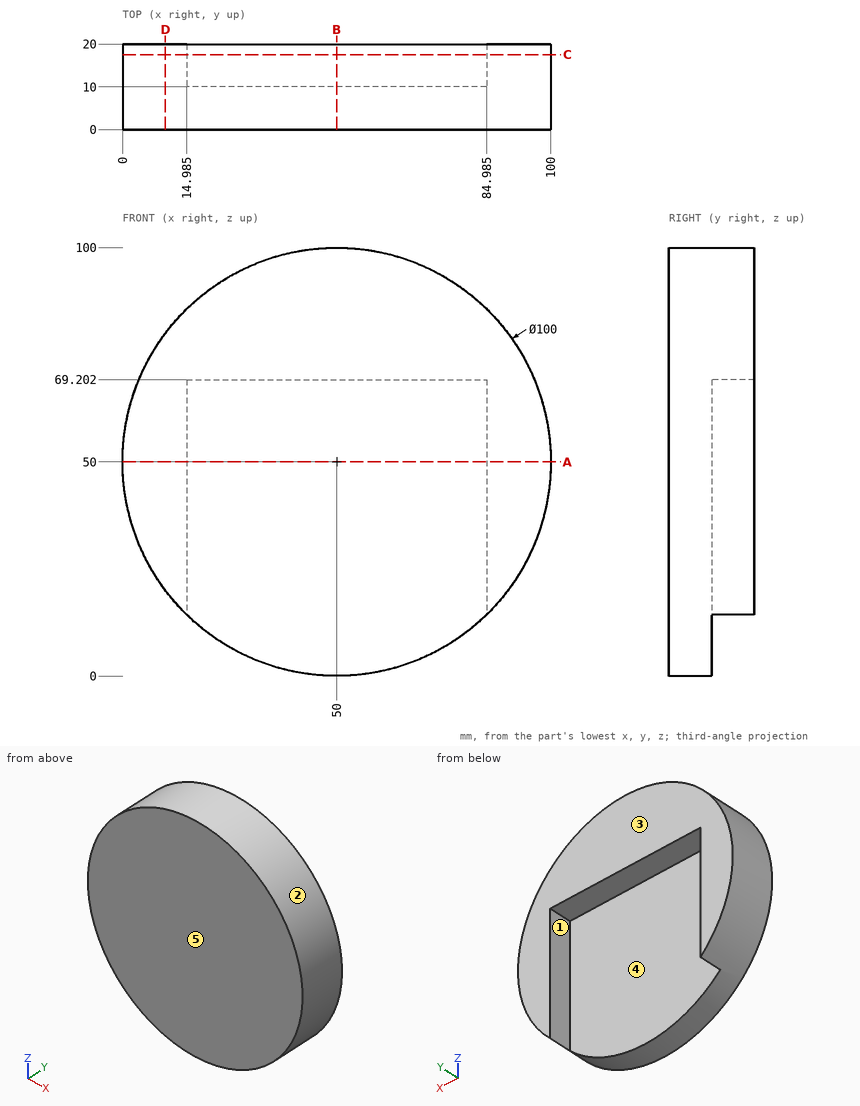
Verification items for this drawing (mm, ordinates from the low corner). A direction names the side the tool comes from. Round coordinates to 2 decimals unless told otherwise and drop trailing zeros. Loops run counter-clockwise (first coordinate to the right, second up) from the corner with the lowest first, then second, coordinate; pieces in that order, holes last. Notation, with made-up numbers: (82.25, 8) -> (98.25, 8) arc R10 ccw to (98.25, 16) -> close; hole circle Ø10 at (40.5, 83.25). An arc over 180 degrees is marked (long way). Write item = value, one per line. Start each with the question number.
1) Thickness scan on probe 1 along Y at (x, z) = (71, 34); probe 2 along X at (y, z) = (12.25, 17.5) (1 decimal); probe 3 along X at (y, z) = (5.75, 47.5). Record the ranges inside material, lowest first.
2) Sectioned sample at A-A, the plane z = 50. Record the cut outline in (x, y) (1 decimal), plus the area to 3 significant figures.
3) Gauge pin test, flat ends, axial feed: pin 1 Ø3 at (y, z) = (15, 45.5) entering from +X; pin 2 Ø8 at (y, z) = (14, 41.5) entering from -X; pin 3 Ø4 at (x, y) = (11, 15) entering from +Z. Record the tip position at first contact, or that the pin passes through.
4) Set-up check for the marked faces 4 and 5: record each of +Z, -Z, +X, -X, +Y, -Y from which the full face is reachable in a straight line by a thin tool's end or side.
5) Sectioned sample at D-D, the plane x = 10. Record the cut outline in (y, z).
6) Sectioned sample at C-C, the plane y = 17.5. Record the cut outline in (x, z) (1 decimal), plus the area to 3 significant figures.
7) Sectioned sample at B-B, the plane x = 50. Record the cut outline in (y, z), plus the area to 3 significant figures.
8) Release check for a two-part mould opening along X. For the marked faces 1, 2 and 3 record: released by +X, released by -X, zero draft, split by the parting line, or undercut.
Results are:
q1.probe_1 = 0 to 10
q1.probe_2 = 12 to 15, 85 to 88
q1.probe_3 = 0.06 to 99.94
q2.outline = (0, 0) -> (100, 0) -> (100, 20) -> (85, 20) -> (85, 10) -> (15, 10) -> (15, 20) -> (0, 20) -> close
q2.area = 1,300 mm^2
q3.pin_1 = 99.91
q3.pin_2 = 0.2
q3.pin_3 = 83.63
q4.face_4 = -Z, +Y
q4.face_5 = +Z, -Z, +X, -X, -Y
q5.outline = (0, 20) -> (20, 20) -> (20, 80) -> (0, 80) -> close
q6.outline = (15, 14.3) -> (15, 69.2) -> (85, 69.2) -> (85, 14.3) arc R50 ccw (long way) to start
q6.area = 3,320 mm^2
q7.outline = (0, 0) -> (10, 0) -> (10, 69.2) -> (20, 69.2) -> (20, 100) -> (0, 100) -> close
q7.area = 1,310 mm^2
q8.face_1 = undercut
q8.face_2 = split by the parting line
q8.face_3 = zero draft
